from build123d import *

# Parameters (mm, degrees)
SKETCH1_R           = 47.85
BOSS_EXTRUDE1_DEPTH = 6
SKETCH2_R           = 14.235
CUT_EXTRUDE1_DEPTH  = 6
FILLET2_R           = 10


with BuildPart() as part:
    # Sketch1 → Boss-Extrude1 (new body)
    with BuildSketch(Plane.XY):
        Circle(SKETCH1_R)
    extrude(amount=BOSS_EXTRUDE1_DEPTH)

    # Sketch2 → Cut-Extrude1 (cut)
    with BuildSketch(Plane.XY.offset(6)):
        Circle(SKETCH2_R)
    extrude(amount=-CUT_EXTRUDE1_DEPTH, mode=Mode.SUBTRACT)

    # Fillet2
    # the kernel refuses this fillet: 10 mm, written as the material it takes off along each edge
    with BuildSketch(Plane(origin=(0, 0, 0), x_dir=(1, 0, 0), z_dir=(0, -1, 0))) as fillet2_piece_1:
        with BuildLine():
            CenterArc((38.68484861, 10), FILLET2_R, 270, 66.421821522)
            Line((38.68484861, 0), (38.68484861, -0.2))
            Line((38.68484861, -0.2), (47.85, -0.2))
            Line((47.85, -0.2), (48.05, 0))
            ThreePointArc((48.05, 0), (48.05, 3), (48.033303028, 5.92))
            Line((48.033303028, 5.92), (47.85, 6))
        make_face()
    revolve(axis=Axis((0, 0, 0), (0, 0, 1)), mode=Mode.SUBTRACT)


solid = part.part
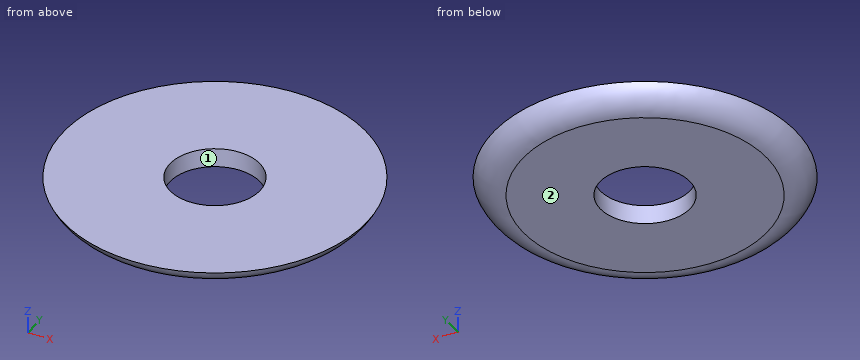
Input: part model. Units: mm. Frame: model coordinates. Face numbers are marked on the shaded views. Give positions to 0.01 mm unless a question says otherwise; leave off trailing zeros. Order: outer loops, then holes, each group sorted by start corner. A loop starts at its lowest first (then second) coordinate and runs counter-clockwise, first axis right, second up.
Q1. Section C-C on z = 3.75. Output: boundary loops of the cut face in (x, y) (3 decimals), and give its area (3 significant figures).
Checked values:
outline: circle Ø92.982 at (0, 0); hole circle Ø28.47 at (0, 0)
area: 6,150 mm2
Q2. Ray query, probe 1 along Y at (x, z) = (-12.5, 2.5); probe 2 along Y at (x, z) = (5, 1.5); probe 3 along X at (y, z) = (-5.5, 2). Return the intervals inside material, ascending.
Checked values:
probe 1: y = -43.54 to -6.81, 6.81 to 43.54
probe 2: y = -43.67 to -13.33, 13.33 to 43.67
probe 3: x = -44.35 to -13.13, 13.13 to 44.35
Q3. Section A-A on y = 0. Output: boundary loops of the cut face in (x, z) (3 decimals), and give its area (3 significant figures).
Checked values:
outline: (-47.85, 6) arc R10 ccw to (-38.685, 0) - (-14.235, 0) - (-14.235, 6) - close; (14.235, 0) - (38.685, 0) arc R10 ccw to (47.85, 6) - (14.235, 6) - close
area: 373 mm2
Q4. Draft query along Y for the marked faces 1 and 2. Return one class per face: +Y half, -Y half, draft (parallel to the pull), parting line (faces both ways), or undercut.
Checked values:
face 1: undercut
face 2: draft
